```python
from build123d import *

# Parameters (mm, degrees)
F0_W     = 203.2
F0_H     = 254
F1_DEPTH = 1.27
F2_R     = 1.27
F3_DEPTH = 3.81
F4_R     = 25.4
F4_W     = 12.7
F4_H     = 38.1
F5_DEPTH = 2.54


with BuildPart() as f1:
    # F0 (on Top) → F1 (new body)
    with BuildSketch(Plane.XY):
        Rectangle(F0_W, F0_H)
    extrude(amount=F1_DEPTH)

    # F2 (on face) → F3 (join)
    with BuildSketch(Plane.XY.offset(1.27)):
        with Locations((-95.25, 120.65)):
            Circle(F2_R)
        with Locations((95.25, 120.65)):
            Circle(F2_R)
        with Locations((95.25, -120.65)):
            Circle(F2_R)
        with Locations((-95.25, -120.65)):
            Circle(F2_R)
    extrude(amount=F3_DEPTH)

    # F4 (on face) → F5 (join)
    with BuildSketch(Plane(origin=(0, 0, 0), x_dir=(1, 0, 0), z_dir=(0, 0, -1))):
        Polygon((-56.228016, 40.367917), (-28.573968, 14.159834), (-19.83794, 23.377851), (-47.491989, 49.585933), align=None)
        Circle(F4_R)
        Polygon((56.228016, 40.367917), (47.491989, 49.585933), (19.83794, 23.377851), (28.573968, 14.159834), align=None)
        with Locations((0.303105, -49.53)):
            Rectangle(F4_W, F4_H)
    extrude(amount=F5_DEPTH)


solid = f1.part
```
Part model, mm, in its own coordinate system. A direction names the side the tool comes from. Round coordinates to 2 decimals unless told otherwise and drop trailing zeros. Order: outer loops, then holes, each group sorted by start corner. A loop starts at its lowest first (then second) coordinate and runs counter-clockwise, first axis right, second up. Notation, with made-up numbers: M 84.25,31 L 116.25,31 A28 cw 116.25,67 Z; hole C 23.5,83 d7. An arc over 180 degrees is marked long. Answer in a Markdown table with one row per item. Add a question column.
Q1. Wall check: L1, parallel to Z at x = -78.5, y = -69; L2, parallel to Z at x = -20, y = -3.5; L3, parallel to X at y = 50, z = -2. Give the ranges that are in metal, low to high. Write a range as from..to.
Q2. Cut at B-B on y = 0. Give the cut face in (x, z).
Q3. Cut at D-D on x = 75. Give the cut face in (y, z), and give its area (3 significant figures).
Q4. Pin check, flat tips, straight feed: pin 1 (1.3 mm diameter, centred on x = 3, z = -1.5, fed in from +Y); pin 2 (1.3 mm diameter, centred on y = 54, z = -2, fed in from +X); pin 3 (0.8 mm diameter, centred on x = 3, z = -1.5, fed in from -Y). Stop position of each tip, or through.
Q5. Cut at C-C on y = -109. Give the cut face in (x, z), and give its area (3 significant figures).
Q6. 3-axis set-ups, long thin cutter, end or side, ignore diameter. For faces 4 (the face through (33.859, -36.665, -1.252)), 5 (the face through (-24.27, -18.7, -1.25)), 6 (the face through (-42.595, -27.447, -1.252)), 7 (the face through (51.921, -44.912, -1.252)): which of +Z, -Z, +X, -X, +Y, -Y reach the whole face in a straight line?
Q7. Mould opens along Y. For faces 1 (the face through (38, -32, -2.54)), 2 (the face through (-5.506, 24.796, -1.252)), 3 (the face through (-51.8, -45.04, -1.25)) say: +Y half, -Y half, draft (parallel to the pull), parting line (faces both ways), or undercut.
Q8. Cut at A-A on x = 0. Give the cut face in (y, z).
Established:
| question | item | result |
|---|---|---|
| 1 | L1 | z = 0..1.27 |
| 1 | L2 | z = -2.54..1.27 |
| 1 | L3 | x = -6.05..6.65 |
| 2 | outline | M -101.6,0 L -25.4,0 L -25.4,-2.54 L 25.4,-2.54 L 25.4,0 L 101.6,0 L 101.6,1.27 L -101.6,1.27 Z |
| 3 | outline | M -127,0 L 127,0 L 127,1.27 L -127,1.27 Z |
| 3 | area | 323 mm2 |
| 4 | pin 1 | stops at y = 68.58 |
| 4 | pin 2 | stops at x = 6.65 |
| 4 | pin 3 | stops at y = -25.27 |
| 5 | outline | M -101.6,0 L 101.6,0 L 101.6,1.27 L -101.6,1.27 Z |
| 5 | area | 258 mm2 |
| 6 | face 4 | -Z, -Y |
| 6 | face 5 | -Z |
| 6 | face 6 | -Z, -X, +Y |
| 6 | face 7 | -Z, +X, -Y |
| 7 | face 1 | draft |
| 7 | face 2 | undercut |
| 7 | face 3 | -Y half |
| 8 | outline | M -127,0 L -25.4,0 L -25.4,-2.54 L 25.4,-2.54 L 25.4,0 L 30.48,0 L 30.48,-2.54 L 68.58,-2.54 L 68.58,0 L 127,0 L 127,1.27 L -127,1.27 Z |
